from build123d import *

# Parameters (mm, degrees)
F0_W     = 55.088852
F0_H     = 40.223607
F0_R     = 6.52573
F1_DEPTH = 25.4
F2_W     = 37.017379
F2_H     = 39.640654
F2_R     = 7.169346
F3_DEPTH = 6.858
F4_W     = 92.106231
F4_H     = 59.752459
F5_DEPTH = 8.382


with BuildPart() as f1:
    # F0 (on Top) → F1 (new body)
    with BuildSketch(Plane.XY):
        with Locations((-27.544426, 6.558197)):
            Rectangle(F0_W, F0_H)
        with Locations((-27.544426, 6.558198)):
            Circle(F0_R, mode=Mode.SUBTRACT)
    extrude(amount=F1_DEPTH)

    # F2 (on Top) → F3 (join)
    with BuildSketch(Plane.XY):
        with Locations((18.508689, 6.558197)):
            Rectangle(F2_W, F2_H)
        with Locations((17.78, 6.558197)):
            Circle(F2_R, mode=Mode.SUBTRACT)
    extrude(amount=F3_DEPTH)

    # F4 (on face) → F5 (join)
    with BuildSketch(Plane(origin=(0, 0, 0), x_dir=(1, 0, 0), z_dir=(0, 0, -1))):
        with Locations((-9.035736, -4.955082)):
            Rectangle(F4_W, F4_H)
    extrude(amount=F5_DEPTH)


solid = f1.part
Verification items for the finished model (mm, model axes). A direction names the side the tool comes from. Round coordinates to 2 decimals unless told otherwise and drop trailing zeros. Loops run counter-clockwise (first coordinate to the right, second up) from the corner with the lowest first, then second, coordinate; pieces in that order, holes last. Notation, with made-up numbers: M 83.25,37.5 L 141.25,37.5 A21 ccw 141.25,65.5 Z; hole C -8,-20.75 d8. An arc over 180 degrees is marked long. Write each question's results on one line, items separated by ' | '.
1) Section check D-D on x = 17.78. Record the boundary of the cut face in (y, z), then the cut area to 3 significant figures.
Checks:
outline: M -24.92,-8.38 L 34.83,-8.38 L 34.83,0 L 26.38,0 L 26.38,6.86 L 13.73,6.86 L 13.73,0 L -0.61,0 L -0.61,6.86 L -13.26,6.86 L -13.26,0 L -24.92,0 Z | area: 674 mm2
2) Scan lines: L1, parallel to Y at x = -34.5, z = 12.5; L2, parallel to Z at x = 32.5, y = 20.5; L3, parallel to Y at x = 17.78, z = 4. Record each from-to range of solid material in increasing order. Write a range as from..to.
Checks:
L1: y = -13.55..26.67 | L2: z = -8.38..6.86 | L3: y = -13.26..-0.61, 13.73..26.38
3) Access from +Z, -Z, +X, -X, +Y, -Y to the whole of each face (thin tool, end or side, straight path). Record for faces 4 (the flat face through (-28, -13.554, 13)), 5 (the flat face through (18, 6, 0)), 6 (the flat face through (18, 26.379, 3)).
Checks:
face 4: +Z, +X, -X, -Y | face 5: +Z | face 6: +Z, +X, +Y
4) Section check B-B on x = -14. Record the boundary of the cut face in (y, z).
Checks:
outline: M -24.92,-8.38 L 34.83,-8.38 L 34.83,0 L 26.67,0 L 26.67,25.4 L -13.55,25.4 L -13.55,0 L -24.92,0 Z
5) Section check C-C on z = 11. Record the boundary of the cut face in (x, y).
Checks:
outline: M -55.09,-13.55 L 0,-13.55 L 0,26.67 L -55.09,26.67 Z; hole C -27.54,6.56 d13.05
6) Mould release check, pull along X, two halves, no side actions. Record for faces 1 (the flat face through (-28, 26.67, 13)), 2 (the flat face through (-55.089, 6, 13)), 3 (the cylindrical face through (24.62, 8.71, 3.38)): released by +X, released by -X, zero draft, split by the parting line, or undercut.
Checks:
face 1: zero draft | face 2: released by -X | face 3: undercut
7) Gauge pin test, flat ends, axial feed: P1, Ø2, axis at x = 20, z = 2.5, coming from the +Y side; P2, Ø6, axis at x = -36, z = 13, coming from the -Y side; P3, Ø4, axis at x = -28, y = 7, coming from the +Z side. Record the tip position at first contact, or that the pin passes through.
Checks:
P1: stops at y = 26.38 | P2: stops at y = -13.55 | P3: stops at z = 0
